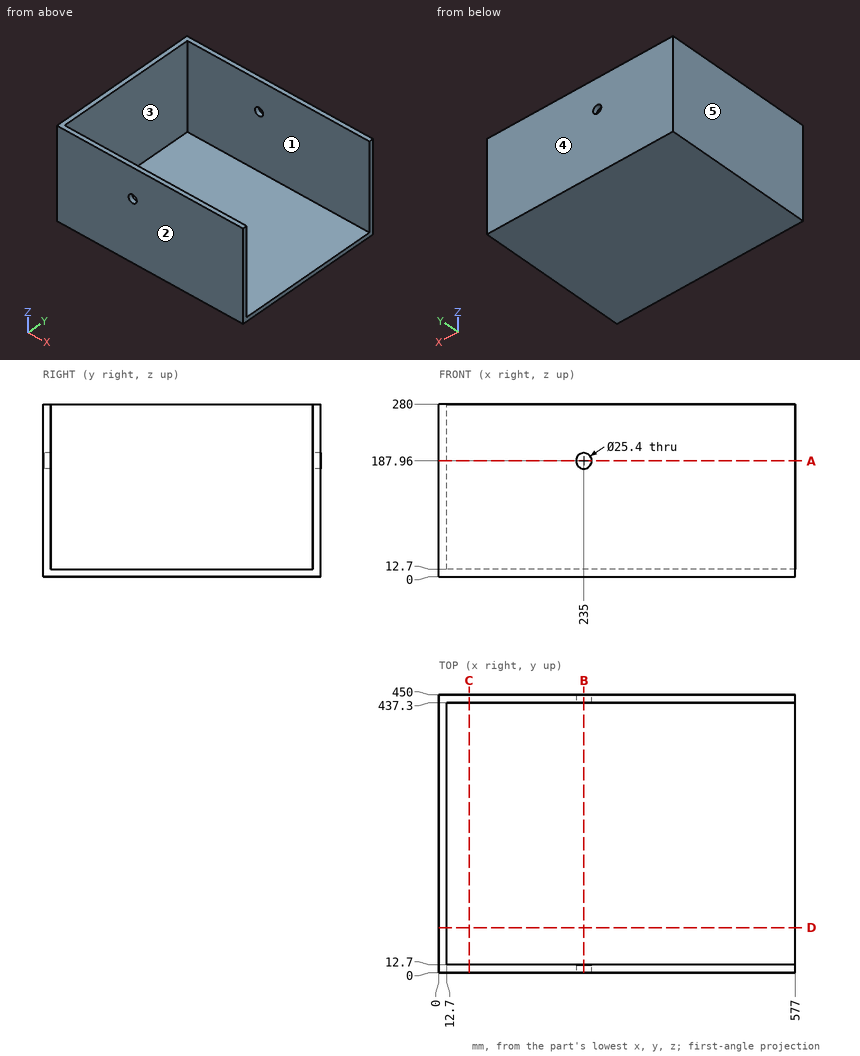
Here's the drawing with two shaded views (mm, measured from the low corner). I have some questions. A direction names the side the tool comes from. Round coordinates to 2 decimals unless told otherwise and drop trailing zeros. Loops run counter-clockwise (first coordinate to the right, second up) from the corner with the lowest first, then second, coordinate; pieces in that order, holes last.
1. If I drill on probe 1 along Z at (x, y) = (235, 3.5); probe 2 along Y at (x, z) = (395, 84); probe 3 along X at (y, z) = (6, 187), over which ranges is the centre line in solid material (lowest first)?
Answers:
probe 1: z = 0 to 175.26, 200.66 to 280
probe 2: y = 0 to 12.7, 437.3 to 450
probe 3: x = 0 to 222.34, 247.66 to 577
2. Suppose I cut it at D-D, the plane y = 73. Please give me the cut outline in (x, z), and give its area (3 significant figures).
Answers:
outline: (0, 0) - (577, 0) - (577, 12.7) - (12.7, 12.7) - (12.7, 280) - (0, 280) - close
area: 10,700 mm2
3. For the marked faces 1 and 2, which set-ups out of +Z, -Z, +X, -X, +Y, -Y let a thin tool reach every point of the face, with its end or its side?
Answers:
face 1: +Z, +X
face 2: +Z, -Z, +X, -X, -Y
4. Will these pins go through, and if not, where does the flat tip stop? pin 1 (23 mm diameter, centred on x = 235, z = 187.96, fed in from +Y); pin 2 (3 mm diameter, centred on y = 100, z = 187.5, fed in from +X).
Answers:
pin 1: passes through
pin 2: stops at x = 12.7
5. Suppose I cut it at B-B, the plane x = 235. Please give me the cut outline in (y, z).
Answers:
outline: (0, 0) - (450, 0) - (450, 175.26) - (437.3, 175.26) - (437.3, 12.7) - (12.7, 12.7) - (12.7, 175.26) - (0, 175.26) - close; (0, 200.66) - (12.7, 200.66) - (12.7, 280) - (0, 280) - close; (437.3, 200.66) - (450, 200.66) - (450, 280) - (437.3, 280) - close
6. Thinking about a two-plate mould opening in Y: for the marked faces 3, 4 and 5, which applies, released by +Y, released by -Y, zero draft, split by the parting line, or undercut?
Answers:
face 3: undercut
face 4: released by +Y
face 5: zero draft
7. Suppose I cut it at C-C, the plane x = 49. Please give me the cut outline in (y, z), and give its area (3 significant figures).
Answers:
outline: (0, 0) - (450, 0) - (450, 280) - (437.3, 280) - (437.3, 12.7) - (12.7, 12.7) - (12.7, 280) - (0, 280) - close
area: 12,500 mm2
8. Suppose I cut it at A-A, the plane z = 187.96. Please give me the cut outline in (x, y), and give its area (3 significant figures).
Answers:
outline: (0, 0) - (222.3, 0) - (222.3, 12.7) - (12.7, 12.7) - (12.7, 437.3) - (222.3, 437.3) - (222.3, 450) - (0, 450) - close; (247.7, 0) - (577, 0) - (577, 12.7) - (247.7, 12.7) - close; (247.7, 437.3) - (577, 437.3) - (577, 450) - (247.7, 450) - close
area: 19,400 mm2
